```python
from build123d import *

# Parameters (mm, degrees)
SKETCH1_R           = 1.65
BOSS_EXTRUDE1_DEPTH = 5
BOSS_EXTRUDE2_DEPTH = 25
SKETCH3_R           = 1.65
CUT_EXTRUDE1_DEPTH  = 31.640005718
SKETCH4_R           = 3.5
CUT_EXTRUDE2_DEPTH  = 2
SKETCH5_R           = 67.5
SKETCH5_R_2         = 66.25
CUT_EXTRUDE3_DEPTH  = 31.0000001


with BuildPart() as part:
    # Sketch1 → Boss-Extrude1 (new body)
    with BuildSketch(Plane(origin=(0, 0, 0), x_dir=(1, 0, 0), z_dir=(0, 1, 0))):
        with BuildLine():
            ThreePointArc((-58.769725256, -31.225340563), (-18.644922026, -63.884813396), (32.748082014, -57.935012077))
            Line((32.748082014, -57.935012077), (-58.769725256, -31.225340563))
        make_face()
        with Locations((-43.522422382, -43.522422382)):
            Circle(SKETCH1_R, mode=Mode.SUBTRACT)
        with Locations((3.221278107, -61.465647864)):
            Circle(SKETCH1_R, mode=Mode.SUBTRACT)
    extrude(amount=BOSS_EXTRUDE1_DEPTH)

    # Sketch2 → Boss-Extrude2 (add)
    with BuildSketch(Plane(origin=(0, 5, 0), x_dir=(1, 0, 0), z_dir=(0, 1, 0))):
        with BuildLine():
            Line((-58.769725256, -31.225340563), (32.748082014, -57.935012077))
            ThreePointArc((32.748082014, -57.935012077), (29.480015366, -59.664320946), (26.120952253, -61.20946294))
            Line((26.120952253, -61.20946294), (-40.494047404, -41.767730103))
            ThreePointArc((-40.494047404, -41.767730103), (-42.54184797, -40.162589972), (-45.131562946, -40.414261085))
            Line((-45.131562946, -40.414261085), (-54.944236671, -37.550410872))
            ThreePointArc((-54.944236671, -37.550410872), (-56.94486731, -34.441030575), (-58.769725256, -31.225340563))
        make_face()
    extrude(amount=BOSS_EXTRUDE2_DEPTH)

    # Sketch3 → Cut-Extrude1 (cut, through all)
    with BuildSketch(Plane(origin=(-14.411642209, 0, 49.379936906), x_dir=(0.959952117, 0, 0.280164118), z_dir=(-0.280164118, 0, 0.959952117))):
        with Locations((41.56355859, 14)):
            Circle(SKETCH3_R)
        with Locations((-24.93644141, 14)):
            Circle(SKETCH3_R)
    extrude(amount=-CUT_EXTRUDE1_DEPTH, mode=Mode.SUBTRACT)

    # Sketch4 → Cut-Extrude2 (cut)
    with BuildSketch(Plane(origin=(-14.411642209, 0, 49.379936906), x_dir=(0.959952117, 0, 0.280164118), z_dir=(-0.280164118, 0, 0.959952117))):
        with Locations((41.56355859, 14)):
            Circle(SKETCH4_R)
        with Locations((-24.93644141, 14)):
            Circle(SKETCH4_R)
    extrude(amount=-CUT_EXTRUDE2_DEPTH, mode=Mode.SUBTRACT)

    # Sketch5 → Cut-Extrude3 (cut, through all)
    with BuildSketch(Plane.XZ):
        Circle(SKETCH5_R)
        Circle(SKETCH5_R_2, mode=Mode.SUBTRACT)
    extrude(amount=-CUT_EXTRUDE3_DEPTH, mode=Mode.SUBTRACT)


solid = part.part
```
Input: part model. Units: mm. Frame: model coordinates. A direction names the side the tool comes from. Round coordinates to 2 decimals unless told otherwise and drop trailing zeros. Loops run counter-clockwise (first coordinate to the right, second up) from the corner with the lowest first, then second, coordinate; pieces in that order, holes last. Notation, with made-up numbers: (-7.75, 68) - (47.25, 68) arc R33 cw to (47.25, 103) - close; hole circle Ø4 at (-28.5, 40.25). An arc over 180 degrees is marked (long way). One line per item, written item: value. Start each with the question number.
(1) Access query for faces 1 (the flat face through (-49.74, 17.32, 39.07)), 2 (the flat face through (-13, 30, 47)), 3 (the cylindrical face through (-42.51, 17.32, 40.17)). Directions: +Z, -Z, +X, -X, +Y, -Y. A direction counts if a zero-diameter tool reaches every point of the face in a straight line with its end or side. Return the directions, or none.
(2) Section B-B, the plane x = -20. Return loops of the section in (y, z).
(3) Contact query for flat-ended pins moving along their axis: P1, Ø4.5, axis at x = 3.22, z = 61.47, coming from the -Y side; P2, Ø5, axis at x = -24, y = 20, coming from the -Z side; P3, Ø6, axis at x = -15, y = 20.5, coming from the -Z side; P4, Ø12, axis at x = -3, y = 15, coming from the +Z side. Output: stop coordinate, or through.
(4) Draft query along X for faces 4 (the cylindrical face through (-17.85, 4.79, 63.8)), 5 (the cylindrical face through (-38.542, 15.115, 38.713)), 6 (the flat face through (-6.951, 17.325, 51.557)). Return one class per face: +X half, -X half, draft (parallel to the pull), parting line (faces both ways), or undercut.
(5) Section A-A, the plane y = 25. Return loops of the section in (x, z), plus the area to 3 significant figures.
(6) Ray query, line 1 (Y direction, x = 11.5, z = 60.5); line 2 (Z direction, x = -15.5, y = 8.5); line 3 (Z direction, x = -4, y = 14). Return the intervals inside material, ascending. Write a range as [from, to].
Results below:
1. face 1: +Z, -X, +Y
1. face 2: +Z, -Z, +X, -X, +Y
1. face 3: +Z, +Y
2. outline: (0, 42.54) - (30, 42.54) - (30, 47.75) - (5, 47.75) - (5, 63.16) - (0, 63.16) - close
3. P1: y = 0
3. P2: z = 40.64
3. P3: z = 43.12
3. P4: z = 54.46
4. face 4: parting line
4. face 5: undercut
4. face 6: -X half
5. outline: (-58.37, 31.34) - (32.35, 57.82) arc R66.25 ccw to (25.67, 61.08) - (-40.49, 41.77) arc R3.5 cw to (-45.13, 40.41) - (-54.49, 37.68) arc R66.25 ccw to start
5. area: 443 mm^2
6. line 1: [0, 5]
6. line 2: [43.85, 49.06]
6. line 3: [47.21, 52.42]
